Here's how the part is built. I have some questions about the finished solid (model axes, mm). A direction names the side the tool comes from. Round coordinates to 2 decimals unless told otherwise and drop trailing zeros. Write each loop counter-clockwise with the first axis right and the second up, starting at its lowest first coordinate (ties: lowest second). Pieces come first, ordered by that corner, then holes. Notation, with made-up numbers: (-39.5, 29) -> (15.5, 29) arc R30 ccw to (15.5, 64) -> close; hole circle Ø4 at (16.5, 71.25). An arc over 180 degrees is marked (long way). Put each result on its own line as item: value. Start each with the question number.
1) If I drill on line 1 along Y through (x, z) = (4.85, 51); line 2 along Y through (x, z) = (5.75, 26.5); line 3 along X through (y, z) = (-9.5, 10), over which ranges is the centre line in solid material (lowest first)? Write a range as [from, to].
2) I want a section at A-A, the plane x = 5.75. List the corners of the cut face in (y, z) for me.
3) We'd pull the mould along X, two halves only. Please class faces 1 (the flat face through (11.35, -5, -2)), 2 (the flat face through (5, -5, 46)), 3 (the flat face through (5, -9.7, 15)): released by +X, released by -X, zero draft, split by the parting line, or undercut.
4) I want a section at C-C, the plane z = 47. List the corners of the cut face in (x, y) for me.
5) I want a section at B-B, the plane y = -5.5. List the corners of the cut face in (x, z) for me, then the cut area to 3 significant figures.
6) Will these pins go through, and if not, where does the flat tip stop? P1, Ø4, axis at x = 2.5, y = -3, coming from the +Z side; P2, Ø1.5, axis at y = -7, z = 15.5, coming from the -X side; P3, Ø3, axis at x = 6.5, z = 18.5, coming from the +Y side; P4, Ø5, axis at y = -9.5, z = 7, coming from the +X side.
7) Which directions (+Z, -Z, +X, -X, +Y, -Y) give clear straight access to the entire face, cutting with the end or side of a thin tool? Please do faces 4 (the flat face through (5, 0, 15)), 5 (the flat face through (9.7, -5, 15)), 6 (the flat face through (0, -5, 15)), 7 (the flat face through (1, -9, 30)), 8 (the flat face through (1, -1, 30)).
8) I want a section at D-D, the plane z = 16. List the corners of the cut face in (x, y) for me.
from build123d import *

# Parameters (mm, degrees)
SKETCH1_W           = 9.7
SKETCH1_H           = 9.7
BOSS_EXTRUDE1_DEPTH = 30
SKETCH2_R           = 4.85
BOSS_EXTRUDE2_DEPTH = 26
SKETCH3_W           = 13
SKETCH3_H           = 13
BOSS_EXTRUDE3_DEPTH = 4
SKETCH4_R           = 3.5
CUT_EXTRUDE1_DEPTH  = 10


with BuildPart() as part:
    # Sketch1 → Boss-Extrude1 (new body)
    with BuildSketch(Plane.XY):
        with Locations((4.85, -4.85)):
            Rectangle(SKETCH1_W, SKETCH1_H)
    extrude(amount=BOSS_EXTRUDE1_DEPTH)

    # Sketch2 → Boss-Extrude2 (add)
    with BuildSketch(Plane.XY.offset(30)):
        with Locations((4.85, -4.85)):
            Circle(SKETCH2_R)
    extrude(amount=BOSS_EXTRUDE2_DEPTH)

    # Sketch3 → Boss-Extrude3 (add)
    with BuildSketch(Plane(origin=(0, 0, 0), x_dir=(-1, 0, 0), z_dir=(0, 0, -1))):
        with Locations((-4.85, -4.85)):
            Rectangle(SKETCH3_W, SKETCH3_H)
    extrude(amount=BOSS_EXTRUDE3_DEPTH)

    # Sketch4 → Cut-Extrude1 (cut)
    with BuildSketch(Plane.XY.offset(56)):
        with Locations((4.85, -4.85)):
            Circle(SKETCH4_R)
    extrude(amount=-CUT_EXTRUDE1_DEPTH, mode=Mode.SUBTRACT)


solid = part.part
Findings:
1. line 1: y = [-9.7, -8.35], [-1.35, 0]
1. line 2: y = [-9.7, 0]
1. line 3: x = [0, 9.7]
2. outline: (-11.35, -4) -> (1.65, -4) -> (1.65, 0) -> (0, 0) -> (0, 30) -> (-0.08, 30) -> (-0.08, 56) -> (-1.47, 56) -> (-1.47, 46) -> (-8.23, 46) -> (-8.23, 56) -> (-9.62, 56) -> (-9.62, 30) -> (-9.7, 30) -> (-9.7, 0) -> (-11.35, 0) -> close
3. face 1: released by +X
3. face 2: undercut
3. face 3: zero draft
4. outline: circle Ø9.7 at (4.85, -4.85); hole circle Ø7 at (4.85, -4.85)
5. outline: (-1.65, -4) -> (11.35, -4) -> (11.35, 0) -> (9.7, 0) -> (9.7, 30) -> (9.66, 30) -> (9.66, 56) -> (8.29, 56) -> (8.29, 46) -> (1.41, 46) -> (1.41, 56) -> (0.04, 56) -> (0.04, 30) -> (0, 30) -> (0, 0) -> (-1.65, 0) -> close
5. area: 524 mm2
6. P1: stops at z = 56
6. P2: stops at x = 0
6. P3: stops at y = 0
6. P4: stops at x = 9.7
7. face 4: +Z, +X, -X, +Y
7. face 5: +Z, +X, +Y, -Y
7. face 6: +Z, -X, +Y, -Y
7. face 7: +Z, -X, -Y
7. face 8: +Z, -X, +Y
8. outline: (0, -9.7) -> (9.7, -9.7) -> (9.7, 0) -> (0, 0) -> close
